```python
from build123d import *

# Parameters (mm, degrees)
F2_DEPTH  = 24
F4_DEPTH  = 24
F5_W      = 74
F5_H      = 699
F6_DEPTH  = 24
F7_R      = 6
F8_DEPTH  = 699.001
F9_SIZE   = 10
F10_W     = 74
F10_H     = 651
F10_H_2   = 24
F10_W_2   = 62
F11_DEPTH = 24
F12_SIZE  = 5


with BuildPart() as f2:
    # F1 (on Front) → F2 (new body)
    with BuildSketch(Plane.XZ):
        Polygon((212.6362921187, 456), (0, 0), (81.6499660032, 0), (259.7794914184, 382), (394.8277852414, 382), (428.2484547083, 0), (502.5311226865, 0), (462.6362921187, 456), align=None)
    extrude(amount=F2_DEPTH)

    # F3 (on face) → F4 (join)
    with BuildSketch(Plane.XZ.offset(24)):
        Polygon((164.6066033287, 353), (199.1133700322, 427), (112.1734633609, 427), (112.1734633609, 353), align=None)
        Polygon((471.6476244618, 353), (465.1734633609, 427), (199.1133700322, 427), (164.6066033287, 353), (246.2565693319, 353), (259.7794914184, 382), (394.8277852414, 382), (397.3649564836, 353), align=None)
        Polygon((419.4995883557, 100), (413.0254272548, 174), (162.7874985222, 174), (128.2807318187, 100), align=None)
        Polygon((162.7874985222, 174), (81.137532519, 174), (46.6307658155, 100), (128.2807318187, 100), align=None)
        Polygon((493.7822563339, 100), (487.308095233, 174), (413.0254272548, 174), (419.4995883557, 100), align=None)
        Polygon((246.2565693319, 353), (397.3649564836, 353), (394.8277852414, 382), (259.7794914184, 382), align=None)
    extrude(amount=F4_DEPTH)

    # F5 (on face) → F6 (join)
    with BuildSketch(Plane.XY.offset(174)):
        with Locations((350.308095233, 301.5)):
            Rectangle(F5_W, F5_H)
    extrude(amount=F6_DEPTH)

    # F7 (on face) → F8 (cut, through all)
    with BuildSketch(Plane.XZ.offset(48)):
        with Locations((149.1734633609, 390)):
            Circle(F7_R)
    extrude(amount=-F8_DEPTH, mode=Mode.SUBTRACT)

    # F9
    f9_edges = [f2.edges().sort_by_distance(p)[0] for p in [
        (112.173463, -36, 427),
        (112.173463, -36, 353),
    ]]
    chamfer(f9_edges, length=F9_SIZE)

    # F10 (on face) → F11 (join)
    with BuildSketch(Plane.XY.offset(456)):
        with Locations((425.6362921187, 325.5)):
            Rectangle(F10_W, F10_H)
        with Locations((331.6362921187, 325.5)):
            Rectangle(F10_W, F10_H)
        with Locations((425.6362921187, -12)):
            Rectangle(F10_W, F10_H_2)
        with Locations((331.6362921187, -12)):
            Rectangle(F10_W, F10_H_2)
        with Locations((243.6362921187, -12)):
            Rectangle(F10_W_2, F10_H_2)
        Polygon((212.6362921187, 0), (274.6362921187, 0), (274.6362921187, 651), (200.6362921187, 651), (200.6362921187, -24), (212.6362921187, -24), align=None)
    extrude(amount=F11_DEPTH)

    # F12
    f12_edges = [f2.edges().sort_by_distance(p)[0] for p in [
        (200.636292, 313.5, 480),
        (462.636292, 313.5, 480),
    ]]
    chamfer(f12_edges, length=F12_SIZE)

    # F13: F2 across face


with BuildPart() as f2_1:
    add(f2.part)
    add(f2.part.mirror(Plane(origin=(350.308095233, 651, 186), x_dir=(-1, 0, 0), z_dir=(0, 1, 0))))


solid = f2_1.part
```
Build history of the part. All positions in model axes, mm. A direction names the side the tool comes from. Round coordinates to 2 decimals unless told otherwise and drop trailing zeros. Write each loop counter-clockwise with the first axis right and the second up, starting at its lowest first coordinate (ties: lowest second). Pieces come first, ordered by that corner, then holes.
1) Band-saw the part on B-B, the plane z = 263.5. List the corners of the cut face in (x, y), and give its area (3 significant figures).
2) Pin check, flat tips, straight feed: pin 1 (22 mm diameter, centred on x = 381.5, y = -14, fed in from +Z); pin 2 (22 mm diameter, centred on x = 443, y = 402, fed in from -Z); pin 3 (15 mm diameter, centred on y = 571, z = 468.5, fed in from +X); pin 4 (5.5 mm diameter, centred on y = 806, z = 461, fed in from -X). Stop position of each tip, or through.
3) Band-saw the part on A-A, the plane y = 200. List the corners of the cut face in (x, z), and give its area (3 significant figures).
4) Mould opens along Z. For faces 1 (the flat face through (331, 642, 456)), 2 (the flat face through (267, 1350, 137)), 3 (the flat face through (465, -12, 0)) say: +Z half, -Z half, draft (parallel to the pull), parting line (faces both ways), or undercut.
5) Band-saw the part on C-C, the plane x = 442. List the corners of the cut face in (y, z), and give its area (3 significant figures).
6) Drill centre lines: probe 1 along Y at (x, z) = (182, 259); probe 2 along Y at (x, z) = (228, 101.5); probe 3 along Z at (x, y) = (367.5, 777.5). Where is each one in solid material? Low to high.
7) 3-axis set-ups, long thin cutter, end or side, ignore diameter. For faces 4 (the flat face through (296, 1338, 427)), 5 (the flat face through (63, -24, 51)), 6 (the flat face through (330, -24, 453)), 7 (the flat face through (460, 1326, 51)), 8 (the flat face through (326, -12, 382)): which of +Z, -Z, +X, -X, +Y, -Y reach the whole face in a straight line?
Ans:
1. outline: (122.87, -24) - (204.52, -24) - (204.52, 0) - (122.87, 0) - close; (122.87, 1302) - (204.52, 1302) - (204.52, 1326) - (122.87, 1326) - close; (405.2, -24) - (479.48, -24) - (479.48, 0) - (405.2, 0) - close; (405.2, 1302) - (479.48, 1302) - (479.48, 1326) - (405.2, 1326) - close
1. area: 7,480 mm2
2. pin 1: stops at z = 480
2. pin 2: stops at z = 456
2. pin 3: stops at x = 462.64
2. pin 4: stops at x = 200.64
3. outline: (200.64, 456) - (274.64, 456) - (274.64, 480) - (205.64, 480) - (200.64, 475) - close; (294.64, 456) - (368.64, 456) - (368.64, 480) - (294.64, 480) - close; (313.31, 174) - (387.31, 174) - (387.31, 198) - (313.31, 198) - close; (388.64, 456) - (462.64, 456) - (462.64, 475) - (457.64, 480) - (388.64, 480) - close
3. area: 7,080 mm2
4. face 1: undercut
4. face 2: draft
4. face 3: -Z half
5. outline: (-48, 100) - (-24, 100) - (-24, 0) - (0, 0) - (0, 456) - (1302, 456) - (1302, 0) - (1326, 0) - (1326, 100) - (1350, 100) - (1350, 174) - (1326, 174) - (1326, 353) - (1350, 353) - (1350, 427) - (1326, 427) - (1326, 480) - (-24, 480) - (-24, 427) - (-48, 427) - (-48, 353) - (-24, 353) - (-24, 174) - (-48, 174) - close
5. area: 61,400 mm2
6. probe 1: y = -24 to 0, 1302 to 1326
6. probe 2: y = -48 to -24, 1326 to 1350
6. probe 3: z = 174 to 198, 456 to 480
7. face 4: +Z, +X, -X, +Y
7. face 5: -Z, +X, -X, -Y
7. face 6: +Z, +X, -X, -Y
7. face 7: -Z, +X, -X, +Y
7. face 8: none
